Read the model definition and answer for the solid it produces. Units are mm, in the model's axes. Face numbers are marked on the shaded views. Coordinates: 2 decimals unless noted, no trailing zeros. Loops run counter-clockwise (first coordinate to the right, second up) from the corner with the lowest first, then second, coordinate; pieces in that order, holes last.
Q1. Straight lines are drawn through the part: line 1 (Y direction, x = -72, z = -2.25); line 2 (Y direction, x = -22.5, z = -2.25); line 3 (Y direction, x = -29, z = -11.75). For each, find the intervals that lie inside material, in ascending order.
Q2. Section A-A (x = -72) is taken. Give the vertices of the cut face in (y, z), then the cut area to 3 significant figures.
Q3. The mould has two halves that part along X. Classify the marked faces 1 and 2: pulls with the +X half, pulls with the -X half, needs draft (parallel to the pull), parting line crosses it, or undercut.
Q4. Section B-B (z = -2.25) is taken. Count the separate pieces of the cut face and the enclosed holes in it, then the cut area to 3 significant figures.
Q5. Section C-C (y = 16.5) is taken. Give the vertices of the cut face in (x, z).
Q6. Flat-ended cylindrical pins translate along their axes: P1, Ø4.5, axis at y = -2.5, z = -7, coming from the +X side; P2, Ø0.5, axis at y = -1.5, z = -11, coming from the +X side; P3, Ø6, axis at y = 12, z = -12.5, coming from the -X side. Find the tip coordinate at first contact, or state that the pin passes through.
from build123d import *

# Parameters (mm, degrees)
SKETCH_R     = 3
PAD_DEPTH    = 15
POCKET_DEPTH = 10.001
CHAMFER_SIZE = 1


with BuildPart() as part:
    # Sketch → Pad (new body)
    with BuildSketch(Plane.XY):
        with BuildLine():
            Line((-30, 10), (-30, 7))
            ThreePointArc((-30, 7), (-29.853553, 6.646447), (-29.5, 6.5))
            Line((-29.5, 6.5), (-28.829405, 6.5))
            ThreePointArc((-28.346442, 6.12941), (-28.525024, 6.396677), (-28.829405, 6.5))
            Line((-28.346442, 6.12941), (-25.908104, -2.97059))
            ThreePointArc((-26.391067, -3.6), (-25.99439, -3.404381), (-25.908104, -2.97059))
            Line((-27.753955, -3.6), (-26.391067, -3.6))
            Line((-29.62941, -3.097473), (-27.753955, -3.6))
            ThreePointArc((-30, -2.61451), (-29.896677, -2.918891), (-29.62941, -3.097473))
            Line((-30, -2.61451), (-30, -1))
            Line((-30, -1), (-31.6, -1))
            Line((-31.6, -1), (-31.6, -3))
            ThreePointArc((-31.6, -3), (-31.228036, -4.095771), (-30.265874, -4.738666))
            Line((-30.265874, -4.738666), (-25.68568, -5.965926))
            ThreePointArc((-25.68568, -5.965926), (-25.557387, -5.991445), (-25.426861, -6))
            Line((-25.426861, -6), (-19.034654, -6))
            ThreePointArc((-19.034654, -6), (-17.817131, -5.586707), (-17.102802, -4.517638))
            Line((-17.102802, -4.517638), (-16.5, -2.267949))
            Line((-16.5, -2.267949), (-16.5, -1.267949))
            Line((-16.5, -1.267949), (-17.5, -1))
            Line((-17.5, -1), (-17.5, 0))
            Line((-17.5, 0), (-16.5, 0))
            Line((-16.5, 0), (-16.5, 6.5))
            ThreePointArc((-15.5, 6.5), (-16, 7), (-16.5, 6.5))
            ThreePointArc((-15.5, 6.5), (-15.06066, 5.43934), (-14, 5))
            Line((-14, 5), (-11.154762, 5))
            ThreePointArc((-10.660644, 4.423529), (-10.775134, 4.825396), (-11.154762, 5))
            Line((-10.660644, 4.423529), (-11.5, -1))
            Line((-11.5, -1), (-11.5, -5))
            ThreePointArc((-11.5, -5), (-11.207107, -5.707107), (-10.5, -6))
            Line((-10.5, -6), (-8.5, -6))
            ThreePointArc((-8.5, -6), (-7.792893, -5.707107), (-7.5, -5))
            Line((-7.5, -5), (-7.5, -1))
            Line((-7.5, -1), (-6.964706, 2.458824))
            ThreePointArc((-4, 5), (-5.952374, 4.27777), (-6.964706, 2.458824))
            Line((-4, 5), (4, 5))
            ThreePointArc((6.964706, 2.458824), (5.952374, 4.27777), (4, 5))
            Line((6.964706, 2.458824), (7.5, -1))
            Line((7.5, -1), (7.5, -5))
            ThreePointArc((7.5, -5), (7.792893, -5.707107), (8.5, -6))
            Line((8.5, -6), (10.5, -6))
            ThreePointArc((10.5, -6), (11.207107, -5.707107), (11.5, -5))
            Line((11.5, -5), (11.5, -1))
            Line((11.5, -1), (10.815406, 3.423529))
            ThreePointArc((11.309524, 4), (10.929896, 3.825396), (10.815406, 3.423529))
            Line((11.309524, 4), (12, 4))
            ThreePointArc((12.5, 3.5), (12.353553, 3.853553), (12, 4))
            Line((12.5, 3.5), (12.5, 2))
            ThreePointArc((12.5, 2), (13.085786, 0.585786), (14.5, 0))
            Line((14.5, 0), (17.5, 0))
            Line((17.5, 0), (17.5, -1.2))
            Line((17.5, -1.2), (15.5, -1.7))
            Line((15.5, -1.7), (15.5, -2.5))
            Line((15.5, -2.5), (17.5, -3))
            Line((17.5, -3), (20.1, -3))
            ThreePointArc((20.1, -3), (20.701412, -2.907434), (21.247153, -2.638304))
            Line((21.247153, -2.638304), (27.272726, 1.580848))
            ThreePointArc((27.272726, 1.580848), (27.586161, 1.938251), (27.69915, 2.4))
            Line((27.69915, 2.4), (27.69915, 5))
            ThreePointArc((28.19915, 5.5), (27.845597, 5.353553), (27.69915, 5))
            Line((34, 5.5), (28.19915, 5.5))
            ThreePointArc((34, 5.5), (34.707107, 5.792893), (35, 6.5))
            Line((35, 6.5), (35, 38))
            ThreePointArc((35, 38), (33.535534, 41.535534), (30, 43))
            Line((-75, 43), (30, 43))
            ThreePointArc((-75, 43), (-78.535534, 41.535534), (-80, 38))
            Line((-80, -7), (-80, 38))
            ThreePointArc((-80, -7), (-78.535534, -10.535534), (-75, -12))
            Line((-41.225519, -12), (-75, -12))
            ThreePointArc((-41.225519, -12), (-37.689985, -10.535534), (-36.225519, -7))
            Line((-36.225519, 10), (-36.225519, -7))
            Line((-30, 10), (-36.225519, 10))
        make_face()
        with Locations((-72, -5)):
            Circle(SKETCH_R, mode=Mode.SUBTRACT)
        with Locations((-72, 11)):
            Circle(SKETCH_R, mode=Mode.SUBTRACT)
        with Locations((-57, 11)):
            Circle(SKETCH_R, mode=Mode.SUBTRACT)
        with Locations((-57, -5)):
            Circle(SKETCH_R, mode=Mode.SUBTRACT)
        with BuildLine():
            Line((-23.894296, -2.758819), (-26.409864, 6.62941))
            ThreePointArc((-26.409864, 6.62941), (-27.022236, 6.982963), (-27.37579, 6.37059))
            Line((-27.37579, 6.37059), (-24.527648, -4.258819))
            ThreePointArc((-24.527648, -4.258819), (-24.170484, -4.793353), (-23.561722, -5))
            Line((-23.561722, -5), (-19.061722, -5))
            ThreePointArc((-19.061722, -5), (-18.452961, -4.793353), (-18.095797, -4.258819))
            Line((-18.095797, -4.258819), (-17.5, -2.035276))
            Line((-17.5, -2.035276), (-18.5, -1.767327))
            Line((-18.5, -1.767327), (-18.5, 1))
            Line((-18.5, 1), (-17.5, 1))
            Line((-17.5, 1), (-17.5, 6.5))
            ThreePointArc((-17.5, 6.5), (-17.646447, 6.853553), (-18, 7))
            Line((-18, 7), (-19.5, 7))
            ThreePointArc((-19.5, 7), (-19.853553, 6.853553), (-20, 6.5))
            Line((-20, 6.5), (-20, -2.5))
            ThreePointArc((-21, -3.5), (-20.292893, -3.207107), (-20, -2.5))
            Line((-21, -3.5), (-22.92837, -3.5))
            ThreePointArc((-23.894296, -2.758819), (-23.537131, -3.293353), (-22.92837, -3.5))
        make_face(mode=Mode.SUBTRACT)
        with BuildLine():
            Line((25.818763, 4), (13.7, 4))
            Line((13.7, 4), (13.7, 2))
            ThreePointArc((13.7, 2), (13.934315, 1.434315), (14.5, 1.2))
            Line((14.5, 1.2), (18.7, 1.2))
            Line((18.7, 1.2), (18.7, -1.8))
            Line((18.7, -1.8), (20.1, -1.8))
            ThreePointArc((20.1, -1.8), (20.400706, -1.753717), (20.673576, -1.619152))
            Line((20.673576, -1.619152), (25.477624, 1.744678))
            ThreePointArc((25.477624, 1.744678), (25.728372, 2.030601), (25.818763, 2.4))
            Line((25.818763, 2.4), (25.818763, 4))
        make_face(mode=Mode.SUBTRACT)
    extrude(amount=-PAD_DEPTH)

    # Sketch001 → Pocket (cut, through all)
    with BuildSketch(Plane.XY.offset(-5)):
        Polygon((-87.346291, -13.915375), (-32.433765, -13.915375), (-32.433765, 9.099434), (44.147678, 9.099434), (44.147678, 52.70644), (-87.346291, 52.70644), align=None)
    extrude(amount=-POCKET_DEPTH, mode=Mode.SUBTRACT)

    # Chamfer
    chamfer_edges = [part.edges().sort_by_distance(p)[0] for p in [
        (-75, 11, 0),
        (-69, 11, -2.5),
        (-75, 11, -5),
        (-60, 11, 0),
        (-54, 11, -2.5),
        (-60, 11, -5),
        (-60, -5, 0),
        (-54, -5, -2.5),
        (-60, -5, -5),
        (-75, -5, 0),
        (-69, -5, -2.5),
        (-75, -5, -5),
    ]]
    chamfer(chamfer_edges, length=CHAMFER_SIZE)


solid = part.part
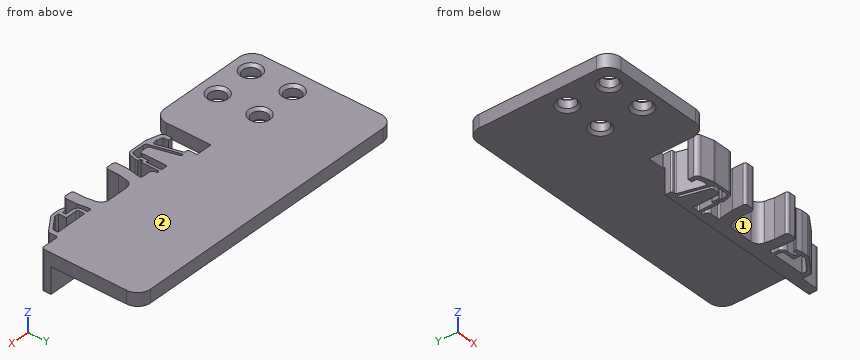
Numbers:
1. line 1: y = -12 to -8, -2 to 8, 14 to 43
1. line 2: y = -6 to -5, -3.5 to 43
1. line 3: y = -5.08 to -3.27, 6.5 to 9.1
2. outline: (-12, -5) - (-9, -5) - (-8, -4) - (-8, -1) - (-9, 0) - (-12, 0) - close; (-2, -4) - (-1, -5) - (7, -5) - (8, -4) - (8, -1) - (7, 0) - (-1, 0) - (-2, -1) - close; (14, -4) - (15, -5) - (43, -5) - (43, 0) - (15, 0) - (14, -1) - close
2. area: 211 mm2
3. face 1: undercut
3. face 2: needs draft
4. separate pieces: 1
4. enclosed holes: 6
4. area: 5,160 mm2
5. outline: (-80, -5) - (35, -5) - (35, 0) - (-80, 0) - close
6. P1: stops at x = 24.66
6. P2: stops at x = 23.23
6. P3: stops at x = -30
